from build123d import *

# Parameters (mm, degrees)
PAD_DEPTH       = 0.8
PAD001_DEPTH    = 10
SKETCH003_R     = 2.8
PAD002_DEPTH    = 9.5
POCKET001_DEPTH = 3
PAD003_DEPTH    = 0.8


with BuildPart() as part:
    # Sketch → Pad (new body)
    with BuildSketch(Plane.XZ):
        with BuildLine():
            Line((-25.5, 13.5), (-25.5, 47.5))
            ThreePointArc((-19.5, 53.5), (-23.742641, 51.742641), (-25.5, 47.5))
            Line((-19.5, 53.5), (19.5, 53.5))
            ThreePointArc((25.5, 47.5), (23.742641, 51.742641), (19.5, 53.5))
            Line((25.5, 47.5), (25.5, 13.5))
            Line((25.5, 13.5), (15.5, 13.5))
            Line((15.5, 13.5), (15.5, 26.5))
            Line((15.5, 26.5), (-15.5, 26.5))
            Line((-15.5, 26.5), (-15.5, 13.5))
            Line((-15.5, 13.5), (-25.5, 13.5))
        make_face()
    extrude(amount=PAD_DEPTH)

    # Sketch001 → Pad001 (join, symmetric)
    with BuildSketch(Plane.YZ):
        Polygon((-1, 26.5), (-7.7, 33.2), (-7.7, 34), (0, 34), (0, 26.5), align=None)
    extrude(amount=PAD001_DEPTH, both=True)

    # Sketch003 (on Face12 of Pad001) → Pad002 (join)
    with BuildSketch(Plane(origin=(0, 0, 34), x_dir=(-1, 0, 0), z_dir=(0, 0, 1))):
        with Locations((0, 4)):
            Circle(SKETCH003_R)
    extrude(amount=-PAD002_DEPTH)

    # Sketch004 → Pocket001 (cut, symmetric)
    with BuildSketch(Plane.YZ):
        Polygon((-1.2, 26.699), (-3.399, 24.5), (-1.2, 24.5), align=None)
        Polygon((-7.7, 30.4), (-7.7, 24.5), (-4.4, 24.5), (-4.4, 27.1), align=None)
    extrude(amount=POCKET001_DEPTH, both=True, mode=Mode.SUBTRACT)

    # Sketch005 (on Face5 of Pocket001) → Pad003 (join)
    with BuildSketch(Plane.XZ.offset(0.8)):
        with BuildLine():
            Line((-7.122628, 52), (-10.327996, 55.205368))
            ThreePointArc((-1.201987, 63.102655), (-10.008916, 64.058239), (-10.327996, 55.205368))
            ThreePointArc((-1.201987, 63.102655), (0, 62.5), (1.201987, 63.102655))
            ThreePointArc((10.327996, 55.205368), (10.008916, 64.058239), (1.201987, 63.102655))
            Line((10.327996, 55.205368), (7.122628, 52))
            Line((7.122628, 52), (-7.122628, 52))
        make_face()
    extrude(amount=-PAD003_DEPTH)


solid = part.part
Input: part model. Units: mm. Frame: model coordinates. A direction names the side the tool comes from. Give positions to 0.01 mm unless a question says otherwise; leave off trailing zeros. Write each loop counter-clockwise with the first axis right and the second up, starting at its lowest first coordinate (ties: lowest second). Pieces come first, ordered by that corner, then holes.
Q1. Pull-direction query (Y, two-part tool) for faces 1 (the face through (0, -5.3, 28)), 2 (the face through (23.789, -0.394, 51.696)), 3 (the face through (-1.95, -6.01, 29)), 4 (the face through (0, 0, 40)); classes: pulls with the +Y half, pulls with the -Y half, needs draft (parallel to the pull), parting line crosses it, or undercut.
Q2. Section C-C, the plane x = 11.5. Output: boundary loops of the cut face in (y, z).
Q3. Section D-D, the plane z = 44. Output: boundary loops of the cut face in (x, y).
Q4. Set-up query: faces 5 (the face through (0, -4, 34)), 6 (the face through (-10, -3, 31)), 7 (the face through (0, -4.4, 26)), 8 (the face through (10, -3, 31)). Return all of +Z, -Z, +X, -X, +Y, -Y with unobstructed straight access to the full face (end or side cutting, diameter ignored); none if empty.
Q5. First-contact query: P1, Ø1, axis at x = -3.5, z = 57, coming from the -Y side; P2, Ø1.1, axis at x = -3.5, y = -0.5, coming from the -Z side; P3, Ø1.3, axis at x = 0.5, z = 26.5, coming from the -Y side. Flat tips, straight axial feed; report the tip coordinate or a pass-through.
Q6. Material intervals for probe 1 along Y at (x, z) = (-1.5, 41.5); probe 2 along X at (y, z) = (-3, 31); probe 3 along Z at (x, y) = (-3, -1.75), sorted ascending.
Q7. Section A-A, the plane z = 19.5. Output: boundary loops of the cut face in (x, y), plus the area to 3 significant figures.
Filled in:
1. face 1: pulls with the -Y half
1. face 2: needs draft
1. face 3: undercut
1. face 4: pulls with the +Y half
2. outline: (-0.8, 26.5) - (0, 26.5) - (0, 53.5) - (-0.8, 53.5) - close; (-0.8, 56.86) - (0, 56.86) - (0, 62.11) - (-0.8, 62.11) - close
3. outline: (-25.5, -0.8) - (25.5, -0.8) - (25.5, 0) - (-25.5, 0) - close
4. face 5: +Z, +X, -X, -Y
4. face 6: +Z, -Z, -X, -Y
4. face 7: -Z, +X, -X, -Y
4. face 8: +Z, -Z, +X, -Y
5. P1: stops at y = -0.8
5. P2: stops at z = 26.5
5. P3: stops at y = -4.45
6. probe 1: y = -0.8 to 0
6. probe 2: x = -10 to 10
6. probe 3: z = 27.25 to 34
7. outline: (-25.5, -0.8) - (-15.5, -0.8) - (-15.5, 0) - (-25.5, 0) - close; (15.5, -0.8) - (25.5, -0.8) - (25.5, 0) - (15.5, 0) - close
7. area: 16.0 mm2
